Verification items for the finished model (mm, model axes). Face numbers are marked on the shaded views. A direction names the side the tool comes from. Coordinates: 2 decimals unless noted, no trailing zeros. Write each loop counter-clockwise with the first axis right and the second up, starting at its lowest first coordinate (ties: lowest second). Pieces come first, ordered by that corner, then holes. Notation, with made-up numbers: M -38,-30 L 1,-30 A20 ccw 1,-24 Z; hole C -29.5,88 d2. An arc over 180 degrees is marked long. Answer in a Markdown table with one row per item.
from build123d import *

# Parameters (mm, degrees)
SKETCH2_R           = 40
BOSS_EXTRUDE2_DEPTH = 5
SKETCH3_R           = 25
CUT_EXTRUDE2_DEPTH  = 8
BOSS_EXTRUDE3_START = 20
SKETCH4_R           = 29
SKETCH4_R_2         = 25
BOSS_EXTRUDE3_DEPTH = 20
BOSS_EXTRUDE4_START = -5
SKETCH5_R           = 2.5
BOSS_EXTRUDE4_DEPTH = 5
CIRPATTERN1_COUNT   = 4


with BuildPart() as part:
    # Sketch2 → Boss-Extrude2 (new body)
    with BuildSketch(Plane.XY):
        Circle(SKETCH2_R)
    extrude(amount=BOSS_EXTRUDE2_DEPTH)

    # Sketch3 → Cut-Extrude2 (cut)
    with BuildSketch(Plane(origin=(0, 0, 0), x_dir=(-1, 0, 0), z_dir=(0, 0, -1))):
        Circle(SKETCH3_R)
    extrude(amount=-CUT_EXTRUDE2_DEPTH, mode=Mode.SUBTRACT)

    # Sketch4 → Boss-Extrude3 (add)
    with BuildSketch(Plane(origin=(0, 0, 0), x_dir=(-1, 0, 0), z_dir=(0, 0, -1)).offset(BOSS_EXTRUDE3_START)):
        with Locations(Location((0, 0, 0), (0, 0, 180))):
            Circle(SKETCH4_R)
        Circle(SKETCH4_R_2, mode=Mode.SUBTRACT)
    extrude(amount=-BOSS_EXTRUDE3_DEPTH)

    # Sketch5 → Boss-Extrude4 (add)
    with BuildSketch(Plane.XY.offset(5).offset(BOSS_EXTRUDE4_START)):
        with BuildLine():
            Line((-5, 39.686269666), (-5, 45))
            ThreePointArc((-5, 45), (0, 50), (5, 45))
            Line((5, 45), (5, 39.686269666))
            ThreePointArc((5, 39.686269666), (0, 40), (-5, 39.686269666))
        make_face()
        with Locations((0, 45)):
            Circle(SKETCH5_R, mode=Mode.SUBTRACT)
    boss_extrude4 = extrude(amount=BOSS_EXTRUDE4_DEPTH)

    # CirPattern1: Boss-Extrude4 ×4 about axis
    cirpattern1_axis = Axis((0, 0, 0), (0, 0, 1))
    for i in range(1, CIRPATTERN1_COUNT):
        add(boss_extrude4.rotate(cirpattern1_axis, i * 360 / CIRPATTERN1_COUNT))


solid = part.part
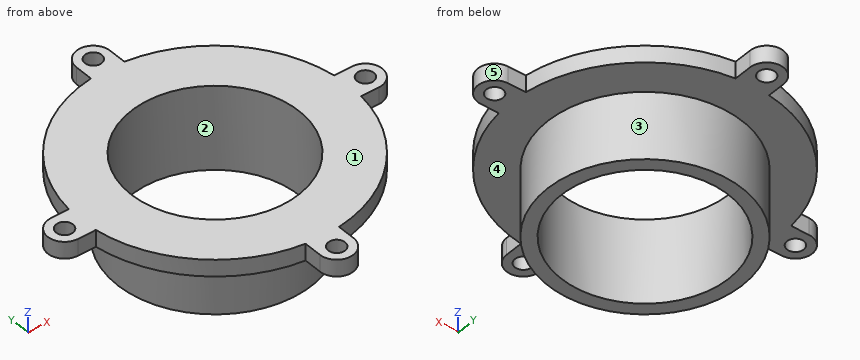
1) Thickness scan on L1, parallel to Y at x = 0, z = 2; L2, parallel to Z at x = -35, y = -11.5; L3, parallel to X at y = 19.5, z = -13.5. Record the ranges inside material, lowest first. Write a range as [from, to].
Response values:
| item | result |
|---|---|
| L1 | y = [-50, -47.5], [-42.5, -25], [25, 42.5], [47.5, 50] |
| L2 | z = [0, 5] |
| L3 | x = [-21.47, -15.64], [15.64, 21.47] |
2) Sectioned sample at A-A (x = 0). Record the cut outline in (y, z), then the cut area to 3 significant figures.
Response values:
| item | result |
|---|---|
| outline | M -50,0 L -47.5,0 L -47.5,5 L -50,5 Z; M -42.5,0 L -29,0 L -29,-20 L -25,-20 L -25,5 L -42.5,5 Z; M 25,-20 L 29,-20 L 29,0 L 42.5,0 L 42.5,5 L 25,5 Z; M 47.5,0 L 50,0 L 50,5 L 47.5,5 Z |
| area | 360 mm² |
3) Release check for a two-part mould opening along X. For the marked faces 1, 2 and 3 record: +X half, -X half, draft (parallel to the pull), parting line (faces both ways), or undercut.
Response values:
| item | result |
|---|---|
| face 1 | draft |
| face 2 | undercut |
| face 3 | parting line |
4) Depth check by flat-ended pin: pin 1 (5.5 mm diameter, centred on x = 42.5, z = 1.5, fed in from +Y); pin 2 (1.5 mm diameter, centred on y = 42.5, z = 1.5, fed in from +X); pin 3 (1.5 mm diameter, centred on y = 43.5, z = 3, fed in from -X). Enter the tip coordinate at first touch or a pass-through.
Response values:
| item | result |
|---|---|
| pin 1 | stops at y = 5 |
| pin 2 | stops at x = 5 |
| pin 3 | stops at x = -5 |
5) Tool access check on the marked faces 4 and 5. Record the directions out of +Z, -Z, +X, -X, +Y, -Y that give a thin tool (end or side, any length) a straight path to the whole face; none if there is none.
Response values:
| item | result |
|---|---|
| face 4 | -Z |
| face 5 | +Z, -Z, +X |
6) Sectioned sample at D-D (x = 19.5). Record the cut outline in (y, z).
Response values:
| item | result |
|---|---|
| outline | M -34.92,0 L -21.47,0 L -21.47,-20 L -15.64,-20 L -15.64,5 L -34.92,5 Z; M 15.64,-20 L 21.47,-20 L 21.47,0 L 34.92,0 L 34.92,5 L 15.64,5 Z |
7) Sectioned sample at B-B (z = 2.25). Record the cut outline in (x, y), then the cut area to 3 significant figures.
Response values:
| item | result |
|---|---|
| outline | M -45,-5 L -39.69,-5 A40 ccw -5,-39.69 L -5,-45 A5 ccw 5,-45 L 5,-39.69 A40 ccw 39.69,-5 L 45,-5 A5 ccw 45,5 L 39.69,5 A40 ccw 5,39.69 L 5,45 A5 ccw -5,45 L -5,39.69 A40 ccw -39.69,5 L -45,5 A5 ccw Z; hole C -45,0 d5; hole C 0,0 d50; hole C 0,-45 d5; hole C 0,45 d5; hole C 45,0 d5 |
| area | 3,350 mm² |
